Input: part model. Units: mm. Frame: model coordinates. A direction names the side the tool comes from. Round coordinates to 2 decimals unless told otherwise and drop trailing zeros. Order: outer loops, then holes, each group sorted by start corner. A loop starts at its lowest first (then second) coordinate and runs counter-clockwise, first axis right, second up.
Item 1: Cut plane B-B on y = -18. Output: boundary loops of the cut face in (x, z), then the cut area to 3 significant figures.
Item 2: Cut plane A-A on x = 16. Output: boundary loops of the cut face in (y, z) (1 decimal).
Item 3: Cut plane D-D on z = 2.8. Output: boundary loops of the cut face in (x, y) (3 decimals), then the cut area to 3 significant figures.
Item 4: Mould query, pull axis X, two halves, no side actions, for faces 1 (the flat face through (22.098, -15, 2)), 2 (the flat face through (0, -31.115, 2)), 3 (the flat face through (33.02, 0, 2)). Classes: released by +X, released by -X, zero draft, split by the parting line, or undercut.
Item 5: Reachability of faces 4 (the flat face through (0, 0, 4.762)), 5 (the flat face through (0, -19.939, 2)) from +Z, -Z, +X, -X, +Y, -Y: full face, straight path, thin tool, end or side. Return the list, or none.
Item 6: Cut plane C-C on x = -16.51. Output: boundary loops of the cut face in (y, z) (1 decimal), then the cut area to 3 significant figures.
Item 7: Line query: L1, parallel to X at y = -27.5, z = 2.8; L2, parallel to X at y = -12, z = 2; L3, parallel to Y at x = -16.51, z = 3.7 (3 decimals). Output: solid intervals per line, ascending.
```python
from build123d import *

# Parameters (mm, degrees)
F1_DEPTH = 4.7625


# Not quite as in the source:
# - a length typed as a fraction of an inch, garbled in the dataset ("3 / 203.2 mm" for 3/8 in), is restored


with BuildPart() as f1:
    # F0 (on Top) → F1 (new body)
    with BuildSketch(Plane.XY):
        with BuildLine():
            Line((22.098, 26.5938), (22.098, 31.115))
            Line((22.098, 31.115), (0, 31.115))
            Line((0, 31.115), (-22.098, 31.115))
            Line((-22.098, 31.115), (-22.098, 26.5938))
            ThreePointArc((-22.098, 26.5938), (-20.6252379961, 25.9837620039), (-20.0152, 24.511))
            ThreePointArc((-20.0152, 24.511), (-20.6252379961, 23.0382379961), (-22.098, 22.4282))
            Line((-22.098, 22.4282), (-22.098, 0.127))
            ThreePointArc((-22.098, 0.127), (-20.8407641431, -0.3937641431), (-20.32, -1.651))
            ThreePointArc((-20.32, -1.651), (-20.8407641431, -2.9082358569), (-22.098, -3.429))
            Line((-22.098, -3.429), (-22.098, -9.779))
            Line((-22.098, -9.779), (22.098, -9.779))
            Line((22.098, -9.779), (22.098, -3.7338))
            ThreePointArc((22.098, -3.7338), (20.0152, -1.651), (22.098, 0.4318))
            Line((22.098, 0.4318), (22.098, 22.4282))
            ThreePointArc((22.098, 22.4282), (20.0152, 24.511), (22.098, 26.5938))
        make_face()
        with BuildLine():
            Line((-22.098, 26.5938), (-22.098, 31.115))
            Line((-22.098, 31.115), (-33.02, 31.115))
            Line((-33.02, 31.115), (-33.02, -31.115))
            Line((-33.02, -31.115), (-22.098, -31.115))
            Line((-22.098, -31.115), (-22.098, -27.559))
            Line((-22.098, -27.559), (-22.098, -19.939))
            Line((-22.098, -19.939), (-22.098, -9.779))
            Line((-22.098, -9.779), (-22.098, -3.429))
            ThreePointArc((-22.098, -3.429), (-23.876, -1.651), (-22.098, 0.127))
            Line((-22.098, 0.127), (-22.098, 22.4282))
            ThreePointArc((-22.098, 22.4282), (-24.1808, 24.511), (-22.098, 26.5938))
        make_face()
        with BuildLine():
            Line((33.02, -27.559), (33.02, 31.115))
            Line((33.02, 31.115), (22.098, 31.115))
            Line((22.098, 31.115), (22.098, 26.5938))
            ThreePointArc((22.098, 26.5938), (23.5707620039, 25.9837620039), (24.1808, 24.511))
            ThreePointArc((24.1808, 24.511), (23.5707620039, 23.0382379961), (22.098, 22.4282))
            Line((22.098, 22.4282), (22.098, 0.4318))
            ThreePointArc((22.098, 0.4318), (23.5707620039, -0.1782379961), (24.1808, -1.651))
            ThreePointArc((24.1808, -1.651), (23.5707620039, -3.1237620039), (22.098, -3.7338))
            Line((22.098, -3.7338), (22.098, -9.779))
            Line((22.098, -9.779), (22.098, -19.939))
            Line((22.098, -19.939), (22.098, -27.559))
            Line((22.098, -27.559), (23.9649, -27.559))
            ThreePointArc((23.9649, -27.559), (26.0477, -25.4762), (28.1305, -27.559))
            Line((28.1305, -27.559), (33.02, -27.559))
        make_face()
        with BuildLine():
            Line((33.02, -31.115), (33.02, -27.559))
            Line((33.02, -27.559), (28.1305, -27.559))
            ThreePointArc((28.1305, -27.559), (26.0477, -29.6418), (23.9649, -27.559))
            Line((23.9649, -27.559), (22.098, -27.559))
            Line((22.098, -27.559), (22.098, -31.115))
            Line((22.098, -31.115), (33.02, -31.115))
        make_face()
        with BuildLine():
            Line((-14.4272, -27.559), (22.098, -27.559))
            Line((22.098, -27.559), (22.098, -19.939))
            Line((22.098, -19.939), (-22.098, -19.939))
            Line((-22.098, -19.939), (-22.098, -27.559))
            Line((-22.098, -27.559), (-18.5928, -27.559))
            ThreePointArc((-18.5928, -27.559), (-16.51, -25.4762), (-14.4272, -27.559))
        make_face()
        with BuildLine():
            Line((-22.098, -31.115), (22.098, -31.115))
            Line((22.098, -31.115), (22.098, -27.559))
            Line((22.098, -27.559), (-14.4272, -27.559))
            ThreePointArc((-14.4272, -27.559), (-16.51, -29.6418), (-18.5928, -27.559))
            Line((-18.5928, -27.559), (-22.098, -27.559))
            Line((-22.098, -27.559), (-22.098, -31.115))
        make_face()
    extrude(amount=F1_DEPTH)


solid = f1.part
```
From the geometry:
1. outline: (-33.02, 0) - (-22.1, 0) - (-22.1, 4.76) - (-33.02, 4.76) - close; (22.1, 0) - (33.02, 0) - (33.02, 4.76) - (22.1, 4.76) - close
1. area: 104 mm2
2. outline: (-31.1, 0) - (-19.9, 0) - (-19.9, 4.8) - (-31.1, 4.8) - close; (-9.8, 0) - (31.1, 0) - (31.1, 4.8) - (-9.8, 4.8) - close
3. outline: (-33.02, -31.115) - (33.02, -31.115) - (33.02, 31.115) - (-33.02, 31.115) - close; hole circle Ø4.166 at (-22.098, 24.511); hole circle Ø3.556 at (-22.098, -1.651); hole (-22.098, -19.939) - (22.098, -19.939) - (22.098, -9.779) - (-22.098, -9.779) - close; hole circle Ø4.166 at (-16.51, -27.559); hole circle Ø4.166 at (22.098, -1.651); hole circle Ø4.166 at (22.098, 24.511); hole circle Ø4.166 at (26.048, -27.559)
3. area: 3,580 mm2
4. face 1: undercut
4. face 2: zero draft
4. face 3: released by +X
5. face 4: +Z, +X, -X, +Y, -Y
5. face 5: +Z, -Z
6. outline: (-31.1, 0) - (-29.6, 0) - (-29.6, 4.8) - (-31.1, 4.8) - close; (-25.5, 0) - (-19.9, 0) - (-19.9, 4.8) - (-25.5, 4.8) - close; (-9.8, 0) - (31.1, 0) - (31.1, 4.8) - (-9.8, 4.8) - close
6. area: 228 mm2
7. L1: x = -33.02 to -18.59, -14.43 to 23.97, 28.13 to 33.02
7. L2: x = -33.02 to -22.1, 22.1 to 33.02
7. L3: y = -31.115 to -29.642, -25.476 to -19.939, -9.779 to 31.115
